from build123d import *

# Parameters (mm, degrees)
BOSS_EXTRUDE1_DEPTH            = 1.3
SKETCH2_W                      = 7
SKETCH2_H                      = 7
CUT_EXTRUDE1_DEPTH             = 8.5
F_2_2_2_2_DIAMETER_HOLE1_D     = 2.2
F_2_2_2_2_DIAMETER_HOLE1_DEPTH = 13
SKETCH18_R                     = 1.5
CUT_EXTRUDE2_DEPTH             = 2.3
SKETCH19_W                     = 0.1
SKETCH19_H                     = 82.2
SKETCH19_W_2                   = 82.2
SKETCH19_H_2                   = 0.1
CUT_EXTRUDE3_DEPTH             = 2.3
CUT_EXTRUDE4_REACH             = 3.3
SKETCH20_R                     = 0.4
SKETCH21_R                     = 0.4
CUT_EXTRUDE5_DEPTH             = 2.3
SKETCH22_R                     = 0.4
CUT_EXTRUDE6_DEPTH             = 2.3
SKETCH23_R                     = 0.4
CUT_EXTRUDE7_DEPTH             = 2.3
SKETCH_1_R                     = 1.9
CUT_EXTRUDE_1_DEPTH            = 0.01
SKETCH_2_R                     = 1.9
CUT_EXTRUDE_2_DEPTH            = 0.01


with BuildPart() as part:
    # Sketch1 → Boss-Extrude1 (new body)
    with BuildSketch(Plane.XY):
        Polygon((-48.1, 12.5), (-43.9, 12.5), (-43.9, -12.5), (-48.1, -12.5), (-48.1, -48.1), (-12.5, -48.1), (-12.5, -43.9), (12.5, -43.9), (12.5, -48.1), (48.1, -48.1), (48.1, -12.5), (43.9, -12.5), (43.9, 12.5), (48.1, 12.5), (48.1, 48.1), (12.5, 48.1), (12.5, 43.9), (-12.5, 43.9), (-12.5, 48.1), (-48.1, 48.1), align=None)
    extrude(amount=BOSS_EXTRUDE1_DEPTH)

    # Sketch2 → Cut-Extrude1 (cut)
    with BuildSketch(Plane.XY.offset(1.3)):
        with Locations((-44.6, 44.6)):
            Rectangle(SKETCH2_W, SKETCH2_H)
        with Locations((44.6, 44.6)):
            Rectangle(SKETCH2_W, SKETCH2_H)
        with Locations((44.6, -44.6)):
            Rectangle(SKETCH2_W, SKETCH2_H)
        with Locations((-44.6, -44.6)):
            Rectangle(SKETCH2_W, SKETCH2_H)
    extrude(amount=-CUT_EXTRUDE1_DEPTH, mode=Mode.SUBTRACT)

    # Ø2.2 (2.2) Diameter Hole1
    with Locations(Plane.XY.offset(1.3)):
        with Locations((-34.5, 45.7), (34.5, 45.7), (-34.5, -45.7), (34.5, -45.7)):
            Hole(F_2_2_2_2_DIAMETER_HOLE1_D / 2, depth=F_2_2_2_2_DIAMETER_HOLE1_DEPTH)

    # Sketch18 → Cut-Extrude2 (cut, through all)
    with BuildSketch(Plane(origin=(0, 0, 0), x_dir=(-1, 0, 0), z_dir=(0, 0, -1))):
        with Locations((41.1, 41.1)):
            Circle(SKETCH18_R)
        with Locations((-41.1, -41.1)):
            Circle(SKETCH18_R)
    extrude(amount=-CUT_EXTRUDE2_DEPTH, mode=Mode.SUBTRACT)

    # Sketch19 → Cut-Extrude3 (cut, through all)
    with BuildSketch(Plane(origin=(0, 0, 0), x_dir=(-1, 0, 0), z_dir=(0, 0, -1))):
        with Locations((48.05, 0)):
            Rectangle(SKETCH19_W, SKETCH19_H)
        with Locations((0, -48.05)):
            Rectangle(SKETCH19_W_2, SKETCH19_H_2)
        with Locations((-48.05, 0)):
            Rectangle(SKETCH19_W, SKETCH19_H)
        with Locations((0, 48.05)):
            Rectangle(SKETCH19_W_2, SKETCH19_H_2)
    extrude(amount=-CUT_EXTRUDE3_DEPTH, mode=Mode.SUBTRACT)

    # Sketch20 → Cut-Extrude4 (cut, up to next)
    with BuildSketch(Plane.XY.offset(1.3), mode=Mode.PRIVATE) as cut_extrude4_sk1:
        with Locations((26.4, 15)):
            Circle(SKETCH20_R)
    cut_extrude4_tool1 = extrude(cut_extrude4_sk1.sketch, amount=-CUT_EXTRUDE4_REACH, mode=Mode.PRIVATE) & part.part
    add(cut_extrude4_tool1.solids().sort_by_distance((26.4, 15, 1.3))[0], mode=Mode.SUBTRACT)
    # Sketch20 → Cut-Extrude4 (cut, up to next)
    with BuildSketch(Plane.XY.offset(1.3), mode=Mode.PRIVATE) as cut_extrude4_sk2:
        with Locations((26.4, 17)):
            Circle(SKETCH20_R)
    cut_extrude4_tool2 = extrude(cut_extrude4_sk2.sketch, amount=-CUT_EXTRUDE4_REACH, mode=Mode.PRIVATE) & part.part
    add(cut_extrude4_tool2.solids().sort_by_distance((26.4, 17, 1.3))[0], mode=Mode.SUBTRACT)
    # Sketch20 → Cut-Extrude4 (cut, up to next)
    with BuildSketch(Plane.XY.offset(1.3), mode=Mode.PRIVATE) as cut_extrude4_sk3:
        with Locations((26.4, 19)):
            Circle(SKETCH20_R)
    cut_extrude4_tool3 = extrude(cut_extrude4_sk3.sketch, amount=-CUT_EXTRUDE4_REACH, mode=Mode.PRIVATE) & part.part
    add(cut_extrude4_tool3.solids().sort_by_distance((26.4, 19, 1.3))[0], mode=Mode.SUBTRACT)
    # Sketch20 → Cut-Extrude4 (cut, up to next)
    with BuildSketch(Plane.XY.offset(1.3), mode=Mode.PRIVATE) as cut_extrude4_sk4:
        with Locations((26.4, 21)):
            Circle(SKETCH20_R)
    cut_extrude4_tool4 = extrude(cut_extrude4_sk4.sketch, amount=-CUT_EXTRUDE4_REACH, mode=Mode.PRIVATE) & part.part
    add(cut_extrude4_tool4.solids().sort_by_distance((26.4, 21, 1.3))[0], mode=Mode.SUBTRACT)
    # Sketch20 → Cut-Extrude4 (cut, up to next)
    with BuildSketch(Plane.XY.offset(1.3), mode=Mode.PRIVATE) as cut_extrude4_sk5:
        with Locations((26.4, 23)):
            Circle(SKETCH20_R)
    cut_extrude4_tool5 = extrude(cut_extrude4_sk5.sketch, amount=-CUT_EXTRUDE4_REACH, mode=Mode.PRIVATE) & part.part
    add(cut_extrude4_tool5.solids().sort_by_distance((26.4, 23, 1.3))[0], mode=Mode.SUBTRACT)
    # Sketch20 → Cut-Extrude4 (cut, up to next)
    with BuildSketch(Plane.XY.offset(1.3), mode=Mode.PRIVATE) as cut_extrude4_sk6:
        with Locations((26.4, 25)):
            Circle(SKETCH20_R)
    cut_extrude4_tool6 = extrude(cut_extrude4_sk6.sketch, amount=-CUT_EXTRUDE4_REACH, mode=Mode.PRIVATE) & part.part
    add(cut_extrude4_tool6.solids().sort_by_distance((26.4, 25, 1.3))[0], mode=Mode.SUBTRACT)
    # Sketch20 → Cut-Extrude4 (cut, up to next)
    with BuildSketch(Plane.XY.offset(1.3), mode=Mode.PRIVATE) as cut_extrude4_sk7:
        with Locations((26.4, 27)):
            Circle(SKETCH20_R)
    cut_extrude4_tool7 = extrude(cut_extrude4_sk7.sketch, amount=-CUT_EXTRUDE4_REACH, mode=Mode.PRIVATE) & part.part
    add(cut_extrude4_tool7.solids().sort_by_distance((26.4, 27, 1.3))[0], mode=Mode.SUBTRACT)
    # Sketch20 → Cut-Extrude4 (cut, up to next)
    with BuildSketch(Plane.XY.offset(1.3), mode=Mode.PRIVATE) as cut_extrude4_sk8:
        with Locations((26.4, 29)):
            Circle(SKETCH20_R)
    cut_extrude4_tool8 = extrude(cut_extrude4_sk8.sketch, amount=-CUT_EXTRUDE4_REACH, mode=Mode.PRIVATE) & part.part
    add(cut_extrude4_tool8.solids().sort_by_distance((26.4, 29, 1.3))[0], mode=Mode.SUBTRACT)
    # Sketch20 → Cut-Extrude4 (cut, up to next)
    with BuildSketch(Plane.XY.offset(1.3), mode=Mode.PRIVATE) as cut_extrude4_sk9:
        with Locations((26.4, 31)):
            Circle(SKETCH20_R)
    cut_extrude4_tool9 = extrude(cut_extrude4_sk9.sketch, amount=-CUT_EXTRUDE4_REACH, mode=Mode.PRIVATE) & part.part
    add(cut_extrude4_tool9.solids().sort_by_distance((26.4, 31, 1.3))[0], mode=Mode.SUBTRACT)
    # Sketch20 → Cut-Extrude4 (cut, up to next)
    with BuildSketch(Plane.XY.offset(1.3), mode=Mode.PRIVATE) as cut_extrude4_sk10:
        with Locations((26.4, 33)):
            Circle(SKETCH20_R)
    cut_extrude4_tool10 = extrude(cut_extrude4_sk10.sketch, amount=-CUT_EXTRUDE4_REACH, mode=Mode.PRIVATE) & part.part
    add(cut_extrude4_tool10.solids().sort_by_distance((26.4, 33, 1.3))[0], mode=Mode.SUBTRACT)
    # Sketch20 → Cut-Extrude4 (cut, up to next)
    with BuildSketch(Plane.XY.offset(1.3), mode=Mode.PRIVATE) as cut_extrude4_sk11:
        with Locations((26.4, 35)):
            Circle(SKETCH20_R)
    cut_extrude4_tool11 = extrude(cut_extrude4_sk11.sketch, amount=-CUT_EXTRUDE4_REACH, mode=Mode.PRIVATE) & part.part
    add(cut_extrude4_tool11.solids().sort_by_distance((26.4, 35, 1.3))[0], mode=Mode.SUBTRACT)
    # Sketch20 → Cut-Extrude4 (cut, up to next)
    with BuildSketch(Plane.XY.offset(1.3), mode=Mode.PRIVATE) as cut_extrude4_sk12:
        with Locations((26.4, 37)):
            Circle(SKETCH20_R)
    cut_extrude4_tool12 = extrude(cut_extrude4_sk12.sketch, amount=-CUT_EXTRUDE4_REACH, mode=Mode.PRIVATE) & part.part
    add(cut_extrude4_tool12.solids().sort_by_distance((26.4, 37, 1.3))[0], mode=Mode.SUBTRACT)

    # Sketch21 → Cut-Extrude5 (cut, through all)
    with BuildSketch(Plane.XY.offset(1.3)):
        with Locations((11, 41.4)):
            Circle(SKETCH21_R)
        with Locations((9, 41.4)):
            Circle(SKETCH21_R)
        with Locations((7, 41.4)):
            Circle(SKETCH21_R)
        with Locations((5, 41.4)):
            Circle(SKETCH21_R)
        with Locations((3, 41.4)):
            Circle(SKETCH21_R)
        with Locations((1, 41.4)):
            Circle(SKETCH21_R)
        with Locations((-1, 41.4)):
            Circle(SKETCH21_R)
        with Locations((-3, 41.4)):
            Circle(SKETCH21_R)
        with Locations((-5, 41.4)):
            Circle(SKETCH21_R)
        with Locations((-7, 41.4)):
            Circle(SKETCH21_R)
        with Locations((-9, 41.4)):
            Circle(SKETCH21_R)
        with Locations((-11, 41.4)):
            Circle(SKETCH21_R)
    extrude(amount=-CUT_EXTRUDE5_DEPTH, mode=Mode.SUBTRACT)

    # Sketch22 → Cut-Extrude6 (cut, through all)
    with BuildSketch(Plane.XY.offset(1.3)):
        with Locations((41.4, 11)):
            Circle(SKETCH22_R)
        with Locations((41.4, 9)):
            Circle(SKETCH22_R)
        with Locations((41.4, 7)):
            Circle(SKETCH22_R)
        with Locations((41.4, 5)):
            Circle(SKETCH22_R)
        with Locations((41.4, 3)):
            Circle(SKETCH22_R)
        with Locations((41.4, 1)):
            Circle(SKETCH22_R)
        with Locations((41.4, -1)):
            Circle(SKETCH22_R)
        with Locations((41.4, -3)):
            Circle(SKETCH22_R)
        with Locations((41.4, -5)):
            Circle(SKETCH22_R)
        with Locations((41.4, -7)):
            Circle(SKETCH22_R)
        with Locations((41.4, -9)):
            Circle(SKETCH22_R)
        with Locations((41.4, -11)):
            Circle(SKETCH22_R)
    extrude(amount=-CUT_EXTRUDE6_DEPTH, mode=Mode.SUBTRACT)

    # Sketch23 → Cut-Extrude7 (cut, through all)
    with BuildSketch(Plane.XY.offset(1.3)):
        with Locations((11, -41.4)):
            Circle(SKETCH23_R)
        with Locations((9, -41.4)):
            Circle(SKETCH23_R)
        with Locations((7, -41.4)):
            Circle(SKETCH23_R)
        with Locations((5, -41.4)):
            Circle(SKETCH23_R)
        with Locations((3, -41.4)):
            Circle(SKETCH23_R)
        with Locations((1, -41.4)):
            Circle(SKETCH23_R)
        with Locations((-1, -41.4)):
            Circle(SKETCH23_R)
        with Locations((-3, -41.4)):
            Circle(SKETCH23_R)
        with Locations((-5, -41.4)):
            Circle(SKETCH23_R)
        with Locations((-7, -41.4)):
            Circle(SKETCH23_R)
        with Locations((-9, -41.4)):
            Circle(SKETCH23_R)
        with Locations((-11, -41.4)):
            Circle(SKETCH23_R)
    extrude(amount=-CUT_EXTRUDE7_DEPTH, mode=Mode.SUBTRACT)

    # ｽｹｯﾁ1 → ｶｯﾄ - 押し出し1 (cut)
    with BuildSketch(Plane.XY.offset(1.3)):
        with Locations((34.5, 45.7)):
            Circle(SKETCH_1_R)
    extrude(amount=-CUT_EXTRUDE_1_DEPTH, mode=Mode.SUBTRACT)

    # ｽｹｯﾁ2 → ｶｯﾄ - 押し出し2 (cut)
    with BuildSketch(Plane(origin=(0, 0, 0), x_dir=(-1, 0, 0), z_dir=(0, 0, -1))):
        with Locations((-34.5, 45.7)):
            Circle(SKETCH_2_R)
    extrude(amount=-CUT_EXTRUDE_2_DEPTH, mode=Mode.SUBTRACT)


solid = part.part
Geometry: final body of the model. Coordinates: model frame, mm. Round coordinates to 2 decimals unless told otherwise and drop trailing zeros. Put each result on its own line as item: value. Start each with the question number.
Q1. Pull-direction query (Y, two-part tool) for faces 1 (the cylindrical face through (-35.09, 46.63, 0.64)), 2 (the flat face through (36, 46, 1.29)); classes: +Y half, -Y half, draft (parallel to the pull), parting line (faces both ways), or undercut.
Q2. First-contact query: pin 1 (0.6 mm diameter, centred on x = 3.5, z = 0.5, fed in from +Y); pin 2 (0.6 mm diameter, centred on y = 45.5, z = 1, fed in from -X); pin 3 (1 mm diameter, centred on x = -27, y = -16, fed in from -Z); pin 4 (3 mm diameter, centred on x = 34.5, y = 45.7, fed in from +Z). Flat tips, straight axial feed; report the tip coordinate or a pass-through.
Q3. Line query: probe 1 along Y at (x, z) = (11, 1); probe 2 along Y at (x, z) = (44, 1.15); probe 3 along X at (y, z) = (29, 1.1). Output: solid intervals per line, ascending.
Q4. Section A-A on z = 0.95. Give the number of separate pieces and of enclosed holes in the cut face, and give its area (3 significant figures).
Ans:
1. face 1: undercut
1. face 2: draft
2. pin 1: stops at y = 43.9
2. pin 2: stops at x = -41.1
2. pin 3: stops at z = 0
2. pin 4: stops at z = 1.29
3. probe 1: y = -43.9 to -41.8, -41 to 41, 41.8 to 43.9
3. probe 2: y = -41.1 to -12.5, 12.5 to 41.1
3. probe 3: x = -48 to 26, 26.8 to 48
4. separate pieces: 1
4. enclosed holes: 52
4. area: 8,570 mm2
